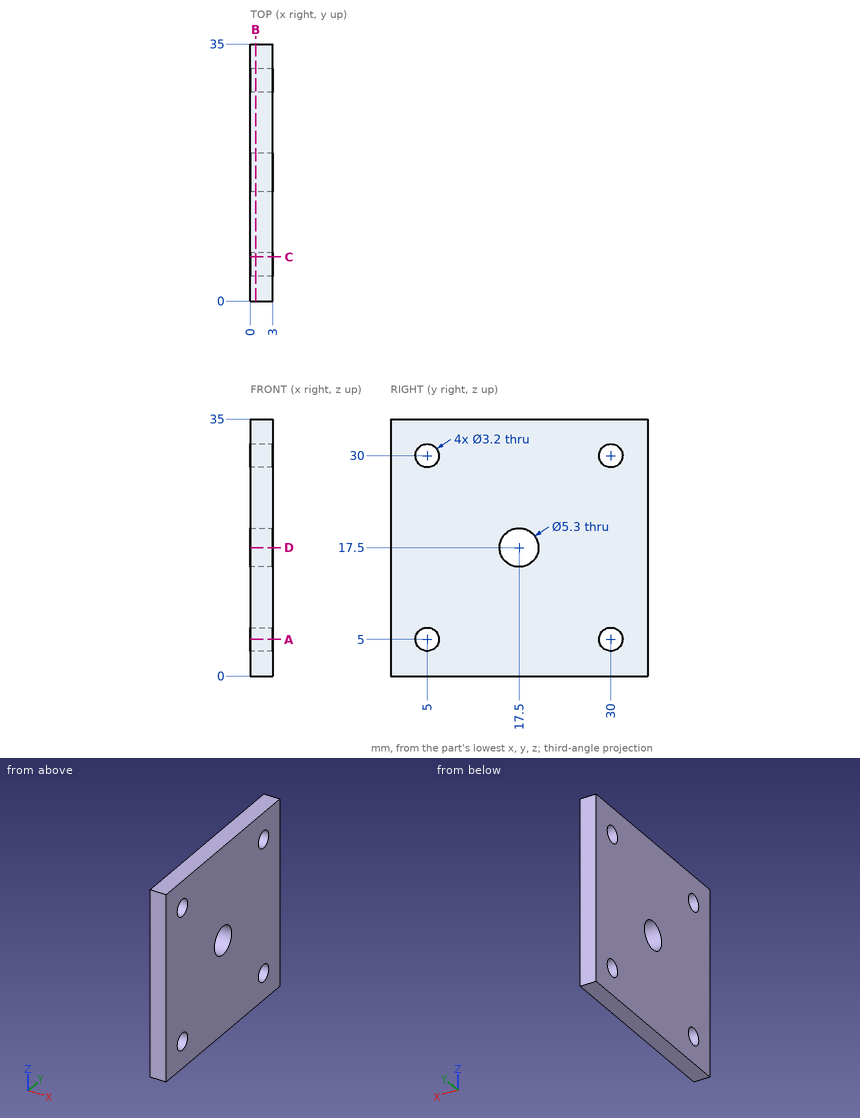
Study the drawing (mm; zero at the part's minimum x, y, z) and answer. Coordinates: 2 decimals unless noted, no trailing zeros. Write each loop counter-clockwise with the first axis right and the second up, starting at its lowest first coordinate (ties: lowest second). Pieces come first, ordered by that corner, then holes. Notation, with made-up numbers: (60.5, 82.5) - (75.5, 82.5) arc R19 cw to (75.5, 107.5) - close; hole circle Ø7 at (23, 22). An arc over 180 degrees is marked (long way). Put each result on its own line as item: value.
1. Find the intervals of material crossed by line 1 along Y through (x, z) = (1.5, 30); line 2 along Y through (x, z) = (0.6, 5.5); line 3 along Y through (x, z) = (1.85, 17.5), in increasing order. Write a range as from..to.
Answer sheet:
line 1: y = 0..3.4, 6.6..28.4, 31.6..35
line 2: y = 0..3.48, 6.52..28.48, 31.52..35
line 3: y = 0..14.85, 20.15..35
2. Flat-ended cylindrical pins translate along their axes: pin 1 Ø4 at (y, z) = (30, 5) entering from +X; pin 2 Ø1.9 at (y, z) = (5, 5) entering from +X. Find the tip coordinate at first contact, or state that the pin passes through.
Answer sheet:
pin 1: stops at x = 3
pin 2: passes through
3. The part is cut by section A-A on z = 5. Give the vertices of the cut face in (x, y), plus the area to 3 significant figures.
Answer sheet:
outline: (0, 0) - (3, 0) - (3, 3.4) - (0, 3.4) - close; (0, 6.6) - (3, 6.6) - (3, 28.4) - (0, 28.4) - close; (0, 31.6) - (3, 31.6) - (3, 35) - (0, 35) - close
area: 85.8 mm^2
4. The part is cut by section C-C on y = 6. Give the vertices of the cut face in (x, z).
Answer sheet:
outline: (0, 0) - (3, 0) - (3, 3.75) - (0, 3.75) - close; (0, 6.25) - (3, 6.25) - (3, 28.75) - (0, 28.75) - close; (0, 31.25) - (3, 31.25) - (3, 35) - (0, 35) - close
5. The part is cut by section B-B on x = 0.7. Give the vertices of the cut face in (y, z), plus the area to 3 significant figures.
Answer sheet:
outline: (0, 0) - (35, 0) - (35, 35) - (0, 35) - close; hole circle Ø3.2 at (5, 5); hole circle Ø3.2 at (5, 30); hole circle Ø5.3 at (17.5, 17.5); hole circle Ø3.2 at (30, 5); hole circle Ø3.2 at (30, 30)
area: 1,170 mm^2
6. The part is cut by section D-D on z = 17.5. Give the vertices of the cut face in (x, y), plus the area to 3 significant figures.
Answer sheet:
outline: (0, 0) - (3, 0) - (3, 14.85) - (0, 14.85) - close; (0, 20.15) - (3, 20.15) - (3, 35) - (0, 35) - close
area: 89.1 mm^2
